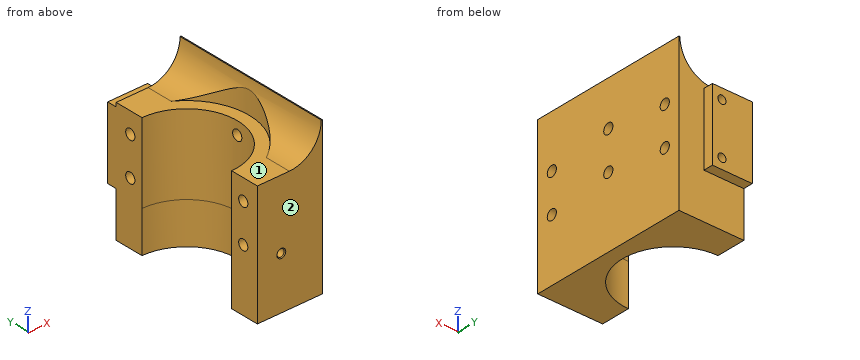
```python
from build123d import *

# Parameters (mm, degrees)
CENTRE_HOLE_FOR_L2_DEPTH      = 40
CENTRE_HOLE_FOR_L2_DEPTH_BACK = 10
SKETCH1_R                     = 39.1
SKETCH1_R_2                   = 31.75
MAIN_STRUCTURE_DEPTH          = 60
MAIN_STRUCTURE_DEPTH_BACK     = 50
SKETCH2_W                     = 100
SKETCH2_H                     = 100
SKETCH2_R                     = 39.1
BEARING_CURVE_DEPTH           = 10
SKETCH6_R                     = 10.5
SHAFT_HOLE_DEPTH              = 10
WRIST_CUTOUT_DEPTH            = 188.082869339
SKETCH11_W                    = 25
SKETCH11_H                    = 45
SKETCH11_R                    = 2.525
BOSS_EXTRUDE1_DEPTH           = 6
CUT_EXTRUDE6_DEPTH            = 168.73789077
CUT_EXTRUDE6_DEPTH_BACK       = 168.73789077
SKETCH18_R                    = 3.25
CUT_EXTRUDE7_START            = -1.5875
CUT_EXTRUDE7_DEPTH            = 1.5875
SKETCH9_R                     = 12.05
BEARING_DEPTH                 = 5
CUT_EXTRUDE8_DEPTH            = 3
SKETCH21_R                    = 3.25
SKETCH21_R_2                  = 1.65
CUT_EXTRUDE9_DEPTH            = 167.868211501
CUT_EXTRUDE10_DEPTH           = 6.35
SKETCH23_R                    = 2.275
CUT_EXTRUDE11_DEPTH           = 6
CHAMFER1_SIZE                 = 0.5
BOSS_EXTRUDE2_DEPTH           = 26


with BuildPart() as part:
    # Sketch1 → Centre Hole for L2 (new, two sides: drawn at the far end of the back side and taken through both)
    with BuildSketch(Plane.XY.offset(-CENTRE_HOLE_FOR_L2_DEPTH_BACK)):
        Circle(SKETCH1_R)
        Circle(SKETCH1_R_2, mode=Mode.SUBTRACT)
    extrude(amount=CENTRE_HOLE_FOR_L2_DEPTH + CENTRE_HOLE_FOR_L2_DEPTH_BACK)

    # Sketch2 → Main Structure (add, two sides: drawn at the far end of the back side and taken through both)
    with BuildSketch(Plane.XY.offset(40).offset(-MAIN_STRUCTURE_DEPTH_BACK)):
        Rectangle(SKETCH2_W, SKETCH2_H)
        Circle(SKETCH2_R, mode=Mode.SUBTRACT)
    extrude(amount=MAIN_STRUCTURE_DEPTH + MAIN_STRUCTURE_DEPTH_BACK)

    # Sketch3 → Bearing Curve (add)
    with BuildSketch(Plane.ZY.offset(50)):
        with BuildLine():
            Line((100, 50), (100, -50))
            ThreePointArc((100, -50), (150, 0), (100, 50))
        make_face()
    bearing_curve = extrude(amount=-BEARING_CURVE_DEPTH)

    # Upright Mirror: Bearing Curve across plane
    add(bearing_curve.mirror(Plane(origin=(0, 0, 0), x_dir=(0, 0, 1), z_dir=(1, 0, 0))))

    # Sketch6 → Shaft Hole (cut)
    with BuildSketch(Plane.ZY.offset(50)):
        with Locations((100, 0)):
            Circle(SKETCH6_R)
    extrude(amount=-SHAFT_HOLE_DEPTH, mode=Mode.SUBTRACT)

    # Sketch4 → Wrist Cutout (cut, through all)
    with BuildSketch(Plane(origin=(0, 50, 0), x_dir=(1, 0, 0), z_dir=(0, 1, 0))):
        with BuildLine():
            Line((-40, -100), (-40, -60))
            ThreePointArc((-40, -60), (-34.142135624, -45.857864376), (-20, -40))
            Line((-20, -40), (20, -40))
            ThreePointArc((20, -40), (34.142135624, -45.857864376), (40, -60))
            Line((40, -60), (40, -100))
            Line((40, -100), (-40, -100))
        make_face()
    extrude(amount=-WRIST_CUTOUT_DEPTH, mode=Mode.SUBTRACT)

    # SurfaceCut1
    split(bisect_by=Plane.ZY, keep=Keep.TOP)

    # Sketch11 → Boss-Extrude1 (add)
    with BuildSketch(Plane(origin=(0, 50, 0), x_dir=(1, 0, 0), z_dir=(0, 1, 0))):
        with Locations((-12.5, -15)):
            Rectangle(SKETCH11_W, SKETCH11_H)
        with Locations(Location((-19, 1, 0), (0, 0, 270))):
            Circle(SKETCH11_R, mode=Mode.SUBTRACT)
        with Locations(Location((-19, -31, 0), (0, 0, 270))):
            Circle(SKETCH11_R, mode=Mode.SUBTRACT)
    extrude(amount=BOSS_EXTRUDE1_DEPTH)

    # Sketch18 → Cut-Extrude6 (cut, two sides: drawn at the far end of the back side and taken through both)
    with BuildSketch(Plane.ZY.offset(50).offset(-CUT_EXTRUDE6_DEPTH_BACK)):
        with Locations((8, 0)):
            Circle(SKETCH18_R)
        with Locations((32, 0)):
            Circle(SKETCH18_R)
    extrude(amount=CUT_EXTRUDE6_DEPTH + CUT_EXTRUDE6_DEPTH_BACK, mode=Mode.SUBTRACT)

    # Sketch19 → Cut-Extrude7 (cut)
    with BuildSketch(Plane(origin=(-40, 0, 0), x_dir=(0, 0, -1), z_dir=(1, 0, 0)).offset(CUT_EXTRUDE7_START)):
        with BuildLine():
            Line((-60, 50), (-100, 50))
            ThreePointArc((-100, 50), (-150, 0), (-100, -50))
            Line((-100, -50), (-60, -50))
            Line((-60, -50), (-60, 50))
        make_face()
    extrude(amount=CUT_EXTRUDE7_DEPTH, mode=Mode.SUBTRACT)

    # Sketch9 → Bearing (cut)
    with BuildSketch(Plane(origin=(-41.5875, 0, 0), x_dir=(0, 0, -1), z_dir=(1, 0, 0))):
        with Locations((-100, 0)):
            Circle(SKETCH9_R)
    extrude(amount=-BEARING_DEPTH, mode=Mode.SUBTRACT)

    # Sketch20 → Cut-Extrude8 (cut)
    with BuildSketch(Plane.ZY.offset(50)):
        with BuildLine():
            Line((-10, -50), (100, -50))
            ThreePointArc((100, -50), (150, 0), (100, 50))
            Line((100, 50), (-10, 50))
            Line((-10, 50), (-10, -50))
        make_face()
    extrude(amount=-CUT_EXTRUDE8_DEPTH, mode=Mode.SUBTRACT)

    # Sketch21 → Cut-Extrude9 (cut, through all)
    with BuildSketch(Plane.ZY.offset(47)):
        with Locations((3, -40)):
            Circle(SKETCH21_R)
        with Locations((27, -40)):
            Circle(SKETCH21_R)
        with Locations(Location((27, 40, 0), (0, 0, 180))):
            Circle(SKETCH21_R)
        with Locations(Location((3, 40, 0), (0, 0, 180))):
            Circle(SKETCH21_R)
        with Locations((125, 0)):
            Circle(SKETCH21_R_2)
    extrude(amount=-CUT_EXTRUDE9_DEPTH, mode=Mode.SUBTRACT)

    # Sketch22 → Cut-Extrude10 (cut)
    with BuildSketch(Plane.ZY.offset(47)):
        with BuildLine():
            Line((-10, 50), (-10, -50))
            Line((-10, -50), (100, -50))
            ThreePointArc((100, -50), (150, 0), (100, 50))
            Line((100, 50), (-10, 50))
        make_face()
    extrude(amount=-CUT_EXTRUDE10_DEPTH, mode=Mode.SUBTRACT)

    # Sketch23 → Cut-Extrude11 (cut)
    with BuildSketch(Plane(origin=(0, -50, 0), x_dir=(-1, 0, 0), z_dir=(0, -1, 0))):
        with Locations(Location((15, 3.25, 0), (0, 0, 90))):
            Circle(SKETCH23_R)
    extrude(amount=-CUT_EXTRUDE11_DEPTH, mode=Mode.SUBTRACT)

    # Chamfer1
    chamfer1_edges = [part.edges().sort_by_distance(p)[0] for p in [
        (-15, -50, -0.975),
    ]]
    chamfer(chamfer1_edges, length=CHAMFER1_SIZE)


with BuildPart() as body_2:
    # Mirror1: mirrored copy
    add(part.part.mirror(Plane.ZY))

    # Sketch24 → Boss-Extrude2 (add)
    with BuildSketch(Plane(origin=(0, 0, -10), x_dir=(-1, 0, 0), z_dir=(0, 0, -1))):
        with BuildLine():
            Line((-40.65, 50), (-40.65, -50))
            Line((-40.65, -50), (0, -50))
            Line((0, -50), (0, -31.75))
            ThreePointArc((0, -31.75), (-31.75, 0), (0, 31.75))
            Line((0, 31.75), (0, 50))
            Line((0, 50), (-40.65, 50))
        make_face()
    extrude(amount=BOSS_EXTRUDE2_DEPTH)


solid = body_2.part
```
Build history of the part. All positions in model axes, mm. Face numbers are marked on the shaded views. A direction names the side the tool comes from. Give positions to 0.01 mm unless a question says otherwise; leave off trailing zeros. Loops run counter-clockwise (first coordinate to the right, second up) from the corner with the lowest first, then second, coordinate; pieces in that order, holes last. Notation, with made-up numbers: (77, 25) -> (107, 25) arc R37 cw to (107, 64) -> close; hole circle Ø4 at (-22, 44). An arc over 180 degrees is marked (long way). One line per question, with ' | ' between items. Start each with the question number.
1) Cut at C-C (z = 8). Give the cut face in (x, y), plus the area to 3 significant figures.
2) Cut at A-A (z = 27). Give the cut face in (x, y), plus the area to 3 significant figures.
3) Cut at D-D (x = 15). Give the cut face in (y, z) (3 decimals).
4) 3-axis set-ups, long thin cutter, end or side, ignore diameter. For the marked faces 1 and 2: which of +Z, -Z, +X, -X, +Y, -Y reach the whole face in a straight line?
5) Probe L1, parallel to Z at x = 13, y = 40; L2, parallel to Z at x = 25, y = 40; L3, parallel to Y at x = 32, z = 3. List the from-to ranges inside material, lowest first.
6) Pin check, flat tips, straight feed: pin 1 (6.5 mm diameter, centred on y = 53.5, z = 22, fed in from +X); pin 2 (1.4 mm diameter, centred on x = 14.5, z = -3, fed in from -Y); pin 3 (1.5 mm diameter, centred on x = 29, z = -16, fed in from +Y). Stop position of each tip, or through.
7) Cut at B-B (y = 40). Give the cut face in (x, z).
Return value:
1) outline: (0, -50) -> (40.65, -50) -> (40.65, -3.25) -> (31.58, -3.25) arc R31.75 cw to (0, -31.75) -> close; (0, 31.75) arc R31.75 cw to (31.58, 3.25) -> (40.65, 3.25) -> (40.65, 50) -> (25, 50) -> (25, 56) -> (0, 56) -> close | area: 2,570 mm^2
2) outline: (0, -50) -> (40.65, -50) -> (40.65, -43.25) -> (0, -43.25) -> close; (0, -36.75) -> (40.65, -36.75) -> (40.65, 36.75) -> (0, 36.75) -> (0, 31.75) arc R31.75 cw to (0, -31.75) -> close; (0, 43.25) -> (40.65, 43.25) -> (40.65, 50) -> (25, 50) -> (25, 56) -> (0, 56) -> close | area: 2,100 mm^2
3) outline: (-50, -36) -> (-27.983, -36) -> (-27.983, 40) -> (-50, 40) -> (-50, -0.475) -> (-49.5, -0.975) -> (-44, -0.975) -> (-44, -5.525) -> (-49.5, -5.525) -> (-50, -6.025) -> close; (27.983, -36) -> (50, -36) -> (50, -7.5) -> (56, -7.5) -> (56, 37.5) -> (50, 37.5) -> (50, 40) -> (27.983, 40) -> close; hole circle Ø6.5 at (-40, 3); hole circle Ø6.5 at (-40, 27); hole circle Ø6.5 at (40, 3); hole circle Ø6.5 at (40, 27)
4) face 1: +Z, -X | face 2: +Z, -Z, +X, -X, -Y
5) L1: -36 to -0.25, 6.25 to 23.75, 30.25 to 40 | L2: -36 to -0.25, 6.25 to 23.75, 30.25 to 40.64 | L3: -50 to -43.25, -36.75 to 36.75, 43.25 to 50
6) pin 1: x = 25 | pin 2: y = -44 | pin 3: y = 50
7) outline: (0, -36) -> (40.65, -36) -> (40.65, -0.25) -> (0, -0.25) -> close; (0, 6.25) -> (40.65, 6.25) -> (40.65, 23.75) -> (0, 23.75) -> close; (0, 30.25) -> (40.65, 30.25) -> (40.65, 60) -> (40, 60) arc R20 cw to (20, 40) -> (0, 40) -> close
